The listing builds one solid part. Answer for the finished solid, in the listing's coordinates (mm). A direction names the side the tool comes from. Coordinates: 2 decimals unless noted, no trailing zeros. Order: outer loops, then holes, each group sorted by start corner. A loop starts at its lowest first (then second) coordinate and runs counter-clockwise, first axis right, second up. Notation, with made-up numbers: M 11.5,21.25 L 35.5,21.25 A28 ccw 35.5,39.25 Z; hole C 74.25,26 d7. An arc over 180 degrees is marked long. One line per item, written item: value. Start each with the question number.
Q1. For faces 4 (the cylindrical face through (-14.43, 10.07, 0.6)), 5 (the flat face through (-9, 5, 10)), determine the directions among +Z, -Z, +X, -X, +Y, -Y from which every point of the face is accessible in a straight line to the end or side of a thin tool.
Q2. Determine the mould class of faces 1 (the cylindrical face through (-14.43, 5.6, 10.14)), 2 (the flat face through (-15, 11, 10)), 3 (the flat face through (9, 5, 10)) for opening direction Y: pulls with the +Y half, pulls with the -Y half, needs draft (parallel to the pull), parting line crosses it, or undercut.
Q3. Each of these flat-tipped pins is pushed along its axis until it touches: pin 1 Ø1 at (x, y) = (9.5, -1.5) entering from +Z; pin 2 Ø8 at (x, z) = (-8.5, 8.5) entering from -Y. Where does it stop, or does it pass through?
Q4. The part is cut by section B-B on y = 0. Give the vertices of the cut face in (x, z).
Q5. The part is cut by section A-A on z = 6.5. Give the vertices of the cut face in (x, y).
Q6. The part is cut by section D-D on x = 12. Give the vertices of the cut face in (y, z), then the cut area to 3 significant figures.
Q7. Straight lines are drawn through the part: line 1 along X through (y, z) = (0, 11); line 2 along X through (y, z) = (-2, 6.5); line 3 along Y through (x, z) = (-12.25, 5.25). For each, find the intervals that lie inside material, in ascending order. Write a range as [from, to].
Q8. The part is cut by section C-C on x = 2.75. Give the vertices of the cut face in (y, z).
```python
from build123d import *

# Parameters (mm, degrees)
SKETCH1_R           = 7.5
SKETCH1_R_2         = 5
SKETCH1_W           = 30
SKETCH1_H           = 10
BOSS_EXTRUDE1_DEPTH = 20
FILLET1_R           = 2


with BuildPart() as part:
    # Sketch1 → Boss-Extrude1 (new body)
    with BuildSketch(Plane.XY):
        Circle(SKETCH1_R)
        Circle(SKETCH1_R_2, mode=Mode.SUBTRACT)
        with Locations((0, 10)):
            Rectangle(SKETCH1_W, SKETCH1_H)
    extrude(amount=BOSS_EXTRUDE1_DEPTH)

    # Fillet1
    fillet1_edges = [part.edges().sort_by_distance(p)[0] for p in [
        (-15, 5, 10),
        (15, 5, 10),
        (15, 10, 20),
        (-15, 10, 20),
        (-15, 10, 0),
        (15, 10, 0),
    ]]
    fillet(fillet1_edges, radius=FILLET1_R)


solid = part.part
```
Output:
1. face 4: -Z, -X, +Y, -Y
1. face 5: +Z, -Z, -X
2. face 1: pulls with the -Y half
2. face 2: needs draft
2. face 3: undercut
3. pin 1: passes through
3. pin 2: stops at y = -6
4. outline: M -7.5,0 L -5,0 L -5,20 L -7.5,20 Z; M 5,0 L 7.5,0 L 7.5,20 L 5,20 Z
5. outline: M -15,7 A2 ccw -13,5 L -5.59,5 A7.5 ccw long 5.59,5 L 13,5 A2 ccw 15,7 L 15,15 L -15,15 Z; hole C 0,0 d10
6. outline: M 5,0 L 15,0 L 15,20 L 5,20 Z
6. area: 200 mm^2
7. line 1: x = [-7.5, -5], [5, 7.5]
7. line 2: x = [-7.23, -4.58], [4.58, 7.23]
7. line 3: y = [5, 15]
8. outline: M -6.98,0 L -4.18,0 L -4.18,20 L -6.98,20 Z; M 4.18,0 L 15,0 L 15,20 L 4.18,20 Z
